Autodesk Inventor part; units mm, degrees
ref_plane "YZ Plane" through (0, 0, 0) normal (1, 0, 0) x (0, 1, 0)
ref_plane "XZ Plane" through (0, 0, 0) normal (0, 1, 0) x (-1, 0, 0)
ref_plane "XY Plane" through (0, 0, 0) normal (0, 0, 1) x (1, 0, 0)
sketch "Эскиз1" plane through (0, 0, 0) normal (0, 1, 0) x (-1, 0, 0)
  line L0 (0, 0) -> (-8, 0)
  line L1 (-8, 0) -> (-8, -28)
  line L2 (-8, -28) -> (0, -28)
  line L3 (0, -28) -> (0, 0)
  line L4 (-4, 0) -> (-4, -10)
  line L5 (-4, -10) -> (-4, -20)
  line L6 (-4, -20) -> (-4, -15)
  line L7 (-4, 0) -> (-4, -5)
  circle A0 centre (-4, -5) radius 1.5
  circle A1 centre (-4, -15) radius 1.5
  dimension "d0" = 8
  dimension "d1" = 28
  dimension "d2" = 10
  dimension "d3" = 10
  dimension "d4" = 3
extrude "Выдавливание1" add sketch "Эскиз1" along normal blind 10
chamfer "Фаска1" distance 0.5 angle 45 4 edges at (5.5, 10, -5) (5.5, 10, -15) (5.5, 0, -15) (5.5, 0, -5)
properties part number "Ограничитель"
Check sheet for the modelled part. Datum: model origin and axes. Units: mm. Round coordinates to 2 decimals unless told otherwise and drop trailing zeros. Order: outer loops, then holes, each group sorted by start corner. A loop starts at its lowest first (then second) coordinate and runs counter-clockwise, first axis right, second up.
1) Section check B-B (x = 4). Record the boundary of the cut face in (y, z), and give its area (3 significant figures).
2) Mould release check, pull along X, two halves, no side actions. Record for faces 1 (the flat face through (8, 5, -14)), 2 (the cylindrical face through (2.614, 4.937, -4.425)), 3 (the flat face through (4, 5, -28)): +X half, -X half, draft (parallel to the pull), parting line (faces both ways), or undercut.
3) Section check A-A (z = -15). Record the boundary of the cut face in (x, y).
4) Section check D-D (x = 2.75). Give the number of separate pieces and of enclosed holes in the cut face, and give its area (3 significant figures).
5) Scan lines: line 1 (Z direction, x = 4, y = 7); line 2 (X direction, y = 3.75, z = -15); line 3 (Z direction, x = 3, y = 7.5). Record each from-to range of solid material in increasing order.
6) Section check C-C (y = 8.5). Record the boundary of the cut face in (x, z), and give its area (3 significant figures).
Result:
1. outline: (0, -28) - (10, -28) - (10, -17) - (9.5, -16.5) - (0.5, -16.5) - (0, -17) - close; (0, -13) - (0.5, -13.5) - (9.5, -13.5) - (10, -13) - (10, -7) - (9.5, -6.5) - (0.5, -6.5) - (0, -7) - close; (0, -3) - (0.5, -3.5) - (9.5, -3.5) - (10, -3) - (10, 0) - (0, 0) - close
1. area: 219 mm2
2. face 1: +X half
2. face 2: undercut
2. face 3: draft
3. outline: (0, 0) - (2, 0) - (2.5, 0.5) - (2.5, 9.5) - (2, 10) - (0, 10) - close; (5.5, 0.5) - (6, 0) - (8, 0) - (8, 10) - (6, 10) - (5.5, 9.5) - close
4. separate pieces: 3
4. enclosed holes: 0
4. area: 245 mm2
5. line 1: z = -28 to -16.5, -13.5 to -6.5, -3.5 to 0
5. line 2: x = 0 to 2.5, 5.5 to 8
5. line 3: z = -28 to -16.12, -13.88 to -6.12, -3.88 to 0
6. outline: (0, -28) - (8, -28) - (8, 0) - (0, 0) - close; hole circle Ø3 at (4, -15); hole circle Ø3 at (4, -5)
6. area: 210 mm2
